```python
from build123d import *

# Parameters (mm, degrees)
SKETCH1_W               = 19.05
SKETCH1_H               = 19.05
BOSS_EXTRUDE1_DEPTH     = 120
SKETCH2_W               = 16.65
SKETCH2_H               = 16.65
CUT_EXTRUDE3_DEPTH      = 121.753680068
CUT_EXTRUDE4_DEPTH      = 121.753680068
CUT_EXTRUDE4_DEPTH_BACK = 121.753680068


with BuildPart() as part:
    # Sketch1 → Boss-Extrude1 (new body)
    with BuildSketch(Plane(origin=(0, 0, 0), x_dir=(1, 0, 0), z_dir=(0, 1, 0))):
        Rectangle(SKETCH1_W, SKETCH1_H)
    extrude(amount=BOSS_EXTRUDE1_DEPTH)

    # Sketch2 → Cut-Extrude3 (cut, through all)
    with BuildSketch(Plane(origin=(0, 0, 0), x_dir=(1, 0, 0), z_dir=(0, 1, 0))):
        Rectangle(SKETCH2_W, SKETCH2_H)
    extrude(amount=CUT_EXTRUDE3_DEPTH, mode=Mode.SUBTRACT)

    # Sketch3 → Cut-Extrude4 (cut, two sides: drawn at the far end of the back side and taken through both)
    with BuildSketch(Plane(origin=(0, 0, 0), x_dir=(0, 0, -1), z_dir=(1, 0, 0)).offset(-CUT_EXTRUDE4_DEPTH_BACK)):
        Polygon((-9.525, 120), (9.525, 118.667894232), (9.525, 120), align=None)
        Polygon((9.525, 0), (-9.525, 0), (9.525, 1.332105768), align=None)
    extrude(amount=CUT_EXTRUDE4_DEPTH + CUT_EXTRUDE4_DEPTH_BACK, mode=Mode.SUBTRACT)


solid = part.part
```
Could you check a few things on this model? Use its own coordinates, in mm. A direction names the side the tool comes from. Coordinates: 2 decimals unless noted, no trailing zeros. Order: outer loops, then holes, each group sorted by start corner. A loop starts at its lowest first (then second) coordinate and runs counter-clockwise, first axis right, second up. Notation, with made-up numbers: M 32,-24 L 66,-24 A30 ccw 66,6 Z; hole C 70.25,89.5 d8. An arc over 180 degrees is marked long. Use a Markdown table: item, result. Add a question column.
Q1. I want a section at A-A on x = 2.5. List the corners of the cut face in (y, z) for me (3 decimals), then the cut area to 3 significant figures.
Q2. If I drill on L1, parallel to X at y = 41, z = 3.5 (3 decimals); L2, parallel to Y at x = 7.25, z = 8.5, over which ranges is the centre line in solid material (lowest first)?
Q3. We'd pull the mould along Z, two halves only. Please class faces 1 (the flat face through (9.525, 59, 0)), 2 (the flat face through (-8.6, 0.657, 0.133)), 3 (the flat face through (8.325, 59, 0)): pulls with the +Z half, pulls with the -Z half, needs draft (parallel to the pull), parting line crosses it, or undercut.
Q4. I want a section at B-B on y = 75. List the corners of the cut face in (x, z) for me (3 decimals), then the cut area to 3 significant figures.
Q5. I want a section at C-C on z = 3.5. List the corners of the cut face in (x, y) for me (3 decimals).
Q6. Which directions (+Z, -Z, +X, -X, +Y, -Y) give clear straight access to the entire face, cutting with the end or side of a thin tool? Please do faces 4 (the flat face through (0, 59, 8.325)), 5 (the flat face through (0, 59, 9.525)).
Q7. I'm going to push flat-ended pins straight in: pin 1 (5 mm diameter, centred on x = 3.5, z = -4.5, fed in from +Y); pin 2 (6 mm diameter, centred on x = 6.5, z = -2, fed in from +Y). Where does each tip first touch, or does it pass through?
Checked values:
| question | item | result |
|---|---|---|
| 1 | outline | M 0,9.525 L 0.084,8.325 L 119.916,8.325 L 120,9.525 Z; M 1.248,-8.325 L 1.332,-9.525 L 118.668,-9.525 L 118.752,-8.325 Z |
| 1 | area | 285 mm² |
| 2 | L1 | -9.525 to -8.325, 8.325 to 9.525 |
| 2 | L2 | 0.07 to 119.93 |
| 3 | face 1 | needs draft |
| 3 | face 2 | pulls with the -Z half |
| 3 | face 3 | undercut |
| 4 | outline | M -9.525,-9.525 L 9.525,-9.525 L 9.525,9.525 L -9.525,9.525 Z; hole M -8.325,-8.325 L 8.325,-8.325 L 8.325,8.325 L -8.325,8.325 Z |
| 4 | area | 85.7 mm² |
| 5 | outline | M -9.525,0.421 L -8.325,0.421 L -8.325,119.579 L -9.525,119.579 Z; M 8.325,0.421 L 9.525,0.421 L 9.525,119.579 L 8.325,119.579 Z |
| 6 | face 4 | +Y, -Y |
| 6 | face 5 | +Z, +X, -X, +Y, -Y |
| 7 | pin 1 | through |
| 7 | pin 2 | y = 119.36 |
